Geometry: final body of the model. Coordinates: model frame, mm. A direction names the side the tool comes from. Round coordinates to 2 decimals unless told otherwise and drop trailing zeros. Write each loop counter-clockwise with the first axis right and the second up, starting at its lowest first coordinate (ties: lowest second). Pieces come first, ordered by that corner, then holes. Notation, with made-up numbers: (63, 87.5) - (118, 87.5) arc R22 ccw to (118, 113.5) - close; hole circle Ø11 at (-11.5, -25). An arc over 180 degrees is marked (long way). Use a Markdown table: item, result. Add a question column.
```python
from build123d import *

# Parameters (mm, degrees)
EXTRUDE1_DEPTH     = 15.24
EXTRUDE2_DEPTH     = 1.5875
EXTRUDE2_TAPER     = 1
SKETCH3_R          = 1.27
EXTRUDE3_DEPTH     = 8.89
EXTRUDE3_TAPER     = 0.5
EXTRUDE4_DEPTH     = 16.2400001
CUT_EXTRUDE1_DEPTH = 16.2400001


with BuildPart() as part:
    # Sketch1 → Extrude1 (new body)
    with BuildSketch(Plane.XY):
        Polygon((-2.3241, 0), (2.3241, 0), (2.415646588, 10.4902), (-2.415646588, 10.4902), align=None)
    extrude(amount=EXTRUDE1_DEPTH)

    # Sketch2 → Extrude2 (add)
    with BuildSketch(Plane(origin=(0, 0, 0), x_dir=(-1, 0, 0), z_dir=(0, 0, -1))):
        with BuildLine():
            Line((-1.841041911, 4.423478779), (-1.8669, 3.683))
            Line((-1.8669, 3.683), (-1.841041911, 2.942521221))
            ThreePointArc((-1.841041911, 2.942521221), (0, 1.698625), (1.841041911, 2.942521221))
            Line((1.841041911, 2.942521221), (1.8669, 3.683))
            Line((1.8669, 3.683), (1.841041911, 4.423478779))
            ThreePointArc((1.841041911, 4.423478779), (0, 5.667375), (-1.841041911, 4.423478779))
        make_face()
    extrude(amount=EXTRUDE2_DEPTH, taper=EXTRUDE2_TAPER)

    # Sketch3 → Extrude3 (cut)
    with BuildSketch(Plane.XY.offset(15.24)):
        with Locations((0, 3.683)):
            Circle(SKETCH3_R)
    extrude(amount=-EXTRUDE3_DEPTH, taper=EXTRUDE3_TAPER, mode=Mode.SUBTRACT)

    # Sketch4 → Extrude4 (cut, through all)
    with BuildSketch(Plane(origin=(0, 0, 0), x_dir=(-1, 0, 0), z_dir=(0, 0, -1))):
        Polygon((-1.013720453, 10.4902), (-0.79375, 10.3632), (0.79375, 10.3632), (1.013720453, 10.4902), align=None)
    extrude(amount=-EXTRUDE4_DEPTH, mode=Mode.SUBTRACT)

    # Sketch5 → Cut-Extrude1 (cut, through all)
    with BuildSketch(Plane(origin=(0, 0, 0), x_dir=(-1, 0, 0), z_dir=(0, 0, -1))):
        Polygon((-1.6891, 0), (-2.329690347, 0.640590347), (-2.3241, 0), align=None)
        Polygon((2.3241, 0), (1.6891, 0), (2.329690347, 0.640590347), align=None)
    extrude(amount=-CUT_EXTRUDE1_DEPTH, mode=Mode.SUBTRACT)


solid = part.part
```
1) Pin query (flat end, axial travel): P1, Ø0.8, axis at x = 0, z = 7.5, coming from the +Y side. Return the tip coordinate at first contact, or that it passes through.
2) Set-up query: faces 1 (the flat face through (2, 10.49, 8)), 2 (the conical face through (-0.91, 4.51, 10.73)). Return all of +Z, -Z, +X, -X, +Y, -Y with unobstructed straight access to the full face (end or side cutting, diameter ignored); none if empty.
3) Material intervals for L1, parallel to Y at x = -0.1, z = 5.75; L2, parallel to X at y = 3, z = 11.5; L3, parallel to Z at x = 1.95, y = 9, sorted ascending. Write a range as from..to.
4) Section C-C, the plane y = 8.5. Return the cut outline in (x, z), then the cut area to 3 significant figures.
5) Section A-A, the plane z = 4.75. Return the cut outline in (x, y).
6) Draft query along Y for faces 3 (the flat face through (0, 4, -1.588)), 4 (the flat face through (0, 4, 6.35)), 5 (the flat face through (0, 0, 8)), 6 (the flat face through (0, 10.363, 8)). Return one class per face: released by +Y, released by -Y, zero draft, split by the parting line, or undercut.
7) Section D-D, the plane z = 13.25. Return the cut outline in (x, y), then the cut area to 3 significant figures.
8) Section B-B, the plane z = 9.5. Return the cut outline in (x, y), then the cut area to 3 significant figures.
Output values:
| question | item | result |
|---|---|---|
| 1 | P1 | stops at y = 10.36 |
| 2 | face 1 | +Z, -Z, +X, -X, +Y |
| 2 | face 2 | +Z |
| 3 | L1 | y = 0..10.36 |
| 3 | L2 | x = -2.35..-1.03, 1.03..2.35 |
| 3 | L3 | z = 0..15.24 |
| 4 | outline | (-2.4, 0) - (2.4, 0) - (2.4, 15.24) - (-2.4, 15.24) - close |
| 4 | area | 73.1 mm^2 |
| 5 | outline | (-2.42, 10.49) - (-2.33, 0.64) - (-1.69, 0) - (1.69, 0) - (2.33, 0.64) - (2.42, 10.49) - (1.01, 10.49) - (0.79, 10.36) - (-0.79, 10.36) - (-1.01, 10.49) - close |
| 6 | face 3 | zero draft |
| 6 | face 4 | undercut |
| 6 | face 5 | released by -Y |
| 6 | face 6 | released by +Y |
| 7 | outline | (-2.42, 10.49) - (-2.33, 0.64) - (-1.69, 0) - (1.69, 0) - (2.33, 0.64) - (2.42, 10.49) - (1.01, 10.49) - (0.79, 10.36) - (-0.79, 10.36) - (-1.01, 10.49) - close; hole circle Ø2.51 at (0, 3.68) |
| 7 | area | 44.2 mm^2 |
| 8 | outline | (-2.42, 10.49) - (-2.33, 0.64) - (-1.69, 0) - (1.69, 0) - (2.33, 0.64) - (2.42, 10.49) - (1.01, 10.49) - (0.79, 10.36) - (-0.79, 10.36) - (-1.01, 10.49) - close; hole circle Ø2.44 at (0, 3.68) |
| 8 | area | 44.4 mm^2 |
